```python
from build123d import *

# Parameters (mm, degrees)
BOSS_EXTRUDE1_DEPTH   = 180
SKETCH3_R             = 11.2
CUT_EXTRUDE1_DEPTH    = 17.5
SKETCH11_W            = 1.6
SKETCH11_H            = 1.8
LPATTERN1_COUNT       = 2
LPATTERN1_PITCH       = 60
M6_TAPPED_HOLE1_D     = 5
M6_TAPPED_HOLE1_DEPTH = 27
M6_TAPPED_HOLE1_TIP   = 1.502151548
CUT_EXTRUDE2_DEPTH    = 3
FILLET1_R             = 1


with BuildPart() as part:
    # Sketch1 → Boss-Extrude1 (new body)
    with BuildSketch(Plane(origin=(0, 0, 0), x_dir=(1, 0, 0), z_dir=(0, 1, 0))):
        Polygon((0, 0), (0, 55), (12.5, 55), (12.5, 45), (16.5, 45), (16.5, 10), (12.5, 10), (12.5, 0), align=None)
    extrude(amount=BOSS_EXTRUDE1_DEPTH)

    # Sketch3 → Cut-Extrude1 (cut, through all)
    with BuildSketch(Plane(origin=(16.5, 0, 0), x_dir=(0, 0, -1), z_dir=(1, 0, 0))):
        with Locations((27.5, 80)):
            Circle(SKETCH3_R)
    cut_extrude1 = extrude(amount=-CUT_EXTRUDE1_DEPTH, mode=Mode.SUBTRACT)

    # Sketch11 → Cut-Revolve1 (revolve, cut)
    with BuildSketch(Plane.XY.offset(-27.5)):
        with BuildLine():
            Line((10, 69.15), (12.5, 69.15))
            Line((12.5, 69.15), (12.5, 67.55))
            ThreePointArc((12.5, 67.55), (12.441421356, 67.408578644), (12.3, 67.35))
            Line((12.3, 67.35), (10.2, 67.35))
            ThreePointArc((10.2, 67.35), (10.058578644, 67.408578644), (10, 67.55))
            Line((10, 67.55), (10, 69.15))
        make_face()
        with Locations((15.7, 66.55)):
            Rectangle(SKETCH11_W, SKETCH11_H)
    cut_revolve1 = revolve(axis=Axis((16.5, 80, -27.5), (-1, 0, 0)), mode=Mode.SUBTRACT)

    # LPattern1: Cut-Extrude1, Cut-Revolve1 ×2
    with Locations(*[(0, i * LPATTERN1_PITCH, 0) for i in range(1, LPATTERN1_COUNT)]):
        add(cut_extrude1, mode=Mode.SUBTRACT)
        add(cut_revolve1, mode=Mode.SUBTRACT)

    # M6 Tapped Hole1
    with Locations(Plane.XZ):
        with Locations((6.5, -12.5), (6.5, -42.5)):
            Hole(M6_TAPPED_HOLE1_D / 2, depth=M6_TAPPED_HOLE1_DEPTH)
            with Locations((0, 0, -(M6_TAPPED_HOLE1_DEPTH + M6_TAPPED_HOLE1_TIP / 2))):  # 118° drill point
                Cone(0, M6_TAPPED_HOLE1_D / 2, M6_TAPPED_HOLE1_TIP, mode=Mode.SUBTRACT)

    # Sketch15 → Cut-Extrude2 (cut)
    with BuildSketch(Plane.ZY):
        Polygon((0, 144.75), (-9.5, 146.75), (-9.5, 133.25), (0, 135.25), align=None)
        Polygon((0, 78.8), (-9.5, 80.8), (-9.5, 67.3), (0, 69.3), align=None)
        Polygon((-55, 39.4), (-45.5, 41.4), (-45.5, 27.9), (-55, 29.9), align=None)
    extrude(amount=-CUT_EXTRUDE2_DEPTH, mode=Mode.SUBTRACT)

    # Fillet1
    fillet1_edges = [part.edges().sort_by_distance(p)[0] for p in [
        (14.5, 180, -10),
        (16.5, 180, -27.5),
        (0, 162.375, 0),
        (0, 109.7, -55),
        (12.5, 90, -55),
        (12.5, 90, 0),
        (14.5, 180, -45),
        (12.5, 180, -50),
        (6.25, 180, -55),
        (0, 180, -27.5),
        (6.25, 180, 0),
        (12.5, 180, -5),
        (0, 107.025, 0),
        (0, 34.65, 0),
        (0, 14.95, -55),
    ]]
    fillet(fillet1_edges, radius=FILLET1_R)


solid = part.part
```
Here's how the part is built. I have some questions about the finished solid (model axes, mm). A direction names the side the tool comes from. Give positions to 0.01 mm unless a question says otherwise; leave off trailing zeros. Order: outer loops, then holes, each group sorted by start corner. A loop starts at its lowest first (then second) coordinate and runs counter-clockwise, first axis right, second up. Notation, with made-up numbers: (67.5, 51.25) - (108.5, 51.25) arc R36 ccw to (108.5, 85.25) - close; hole circle Ø6 at (8.5, 20). An arc over 180 degrees is marked (long way). Answer as a JSON object with one key per item and string values. Group by question number.
Item 1: If we section it at C-C on z = -27.5: Give the number of separate pieces and of enclosed holes in the cut face, and give its area (3 significant figures).
Item 2: If we section it at A-A on y = 18: Please give me the cut outline in (x, z).
Item 3: Please list where these lines run through material, in increasing order: probe 1 along Z at (x, y) = (11.5, 80); probe 2 along Y at (x, z) = (8.25, -37); probe 3 along Y at (x, z) = (4.5, -37.5).
Item 4: If we mould it in two halves opening along Z, with no side actions, what happens to faces 1 (the flat face through (1.479, 134.236, -4.816)), 2 (the flat face through (6, 88, -55))? For each: pulls with the +Z half, pulls with the -Z half, needs draft (parallel to the pull), parting line crosses it, or undercut.
Item 5: For P1, Ø2, axis at x = 13, y = 57, coming from the -Z side; P2, Ø3, axis at x = 15.5, y = 65.5, coming from the +Z side; P3, Ø1.5, axis at x = 1.5, y = 140.5, coming from the +Z side, each with a flat end and sliding along its axis, tell me the tip position at first contact or that it passes through.
Item 6: If we section it at B-B on y = 53.5: Please give me the cut outline in (x, z), and give its area (3 significant figures).
Item 7: Which directions (+Z, -Z, +X, -X, +Y, -Y) give clear straight access to the entire face, cutting with the end or side of a thin tool? Please do faces 3 (the cylindrical face through (15.711, 92.538, -26.948)), 4 (the cylindrical face through (7.04, 13.69, -44.94)), 5 (the flat face through (1.479, 145.736, -4.684)), 6 (the flat face through (12.5, 75, -17)).
Result set:
{
 "1": {"separate pieces": "3", "enclosed holes": "0", "area": "2,200 mm²"},
 "2": {"outline": "(0, -54) arc R1 ccw to (1, -55) - (11.5, -55) arc R1 ccw to (12.5, -54) - (12.5, -45) - (16.5, -45) - (16.5, -10) - (12.5, -10) - (12.5, -1) arc R1 ccw to (11.5, 0) - (1, 0) arc R1 ccw to (0, -1) - close; hole circle Ø5 at (6.5, -42.5); hole circle Ø5 at (6.5, -12.5)"},
 "3": {"probe 1": "-55 to -40.15, -14.85 to 0", "probe 2": "0 to 74.07, 85.93 to 134.07, 145.93 to 180", "probe 3": "0 to 74.96, 85.04 to 134.96, 145.04 to 180"},
 "4": {"face 1": "undercut", "face 2": "pulls with the -Z half"},
 "5": {"P1": "z = -54.87", "P2": "z = -10", "P3": "z = -9.5"},
 "6": {"outline": "(0, -54) arc R1 ccw to (1, -55) - (11.5, -55) arc R1 ccw to (12.5, -54) - (12.5, -45) - (16.5, -45) - (16.5, -10) - (12.5, -10) - (12.5, -1) arc R1 ccw to (11.5, 0) - (1, 0) arc R1 ccw to (0, -1) - close", "area": "827 mm²"},
 "7": {"face 3": "+X", "face 4": "-Y", "face 5": "-X", "face 6": "none"}
}
